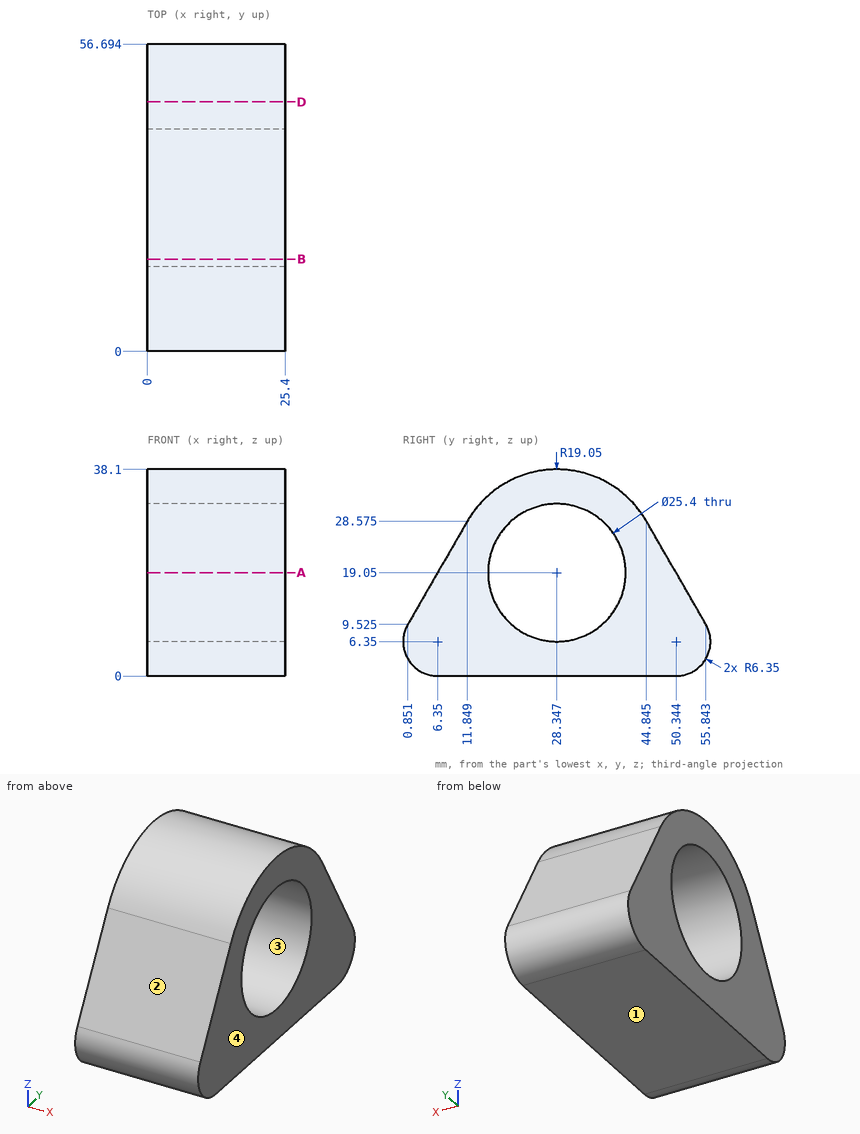
Geometry: see drawing. Coordinates: mm, zero at the bounding-box minimum. Round coordinates to 2 decimals unless told otherwise and drop trailing zeros. Write each loop counter-clockwise with the first axis right and the second up, starting at its lowest first coordinate (ties: lowest second). Pieces come first, ordered by that corner, then holes. Notation, with made-up numbers: M -35.5,1.5 L -17.5,1.5 A13 cw -17.5,5.5 Z; hole C 2.5,45 d9. An arc over 180 degrees is marked long. Answer as a JSON object with one key per item and string values. Group by question number.
(1) Section query B-B on y = 17. Output: boundary loops of the cut face in (x, z), then the cut area to 3 significant figures.
(2) Mould query, pull axis Z, two halves, no side actions, for the marked faces 1, 2, 3 and 4. Classes: +Z half, -Z half, draft (parallel to the pull), parting line (faces both ways), or undercut.
(3) Section query D-D on y = 46. Output: boundary loops of the cut face in (x, z), then the cut area to 3 significant figures.
(4) First-contact query: pin 1 (4 mm diameter, centred on y = 37, z = 21, fed in from +X); pin 2 (3 mm diameter, centred on x = 20.5, z = 24, fed in from -Y); pin 3 (3 mm diameter, centred on x = 21, z = 20, fed in from +Y); pin 4 (3 mm diameter, centred on x = 3.5, z = 31.5, fed in from -Y). Flat tips, straight axial feed; report the tip coordinate or a pass-through.
(5) Section query A-A on z = 19.05. Output: boundary loops of the cut face in (x, y), then the cut area to 3 significant figures.
(6) Ray query, line 1 (Z direction, x = 12.25, y = 21.5) (1 decimal); line 2 (Z direction, x = 12, y = 35); line 3 (Y direction, x = 11.75, z = 25) (1 decimal). Return the intervals inside material, ascending. Write a range as [from, to].
Computed values:
{
 "1": {"outline": "M 0,0 L 25.4,0 L 25.4,13.35 L 0,13.35 Z; M 0,24.75 L 25.4,24.75 L 25.4,34.35 L 0,34.35 Z", "area": "583 mm^2"},
 "2": {"face 1": "-Z half", "face 2": "+Z half", "face 3": "undercut", "face 4": "draft"},
 "3": {"outline": "M 0,0 L 25.4,0 L 25.4,26.57 L 0,26.57 Z", "area": "675 mm^2"},
 "4": {"pin 1": "through", "pin 2": "y = 8.34", "pin 3": "y = 50.66", "pin 4": "y = 12.76"},
 "5": {"outline": "M 0,6.35 L 25.4,6.35 L 25.4,15.65 L 0,15.65 Z; M 0,41.05 L 25.4,41.05 L 25.4,50.34 L 0,50.34 Z", "area": "472 mm^2"},
 "6": {"line 1": "[0, 8.4], [29.7, 36.8]", "line 2": "[0, 8.23], [29.87, 36.9]", "line 3": "[9.8, 17.1], [39.6, 46.9]"}
}
